Can you work these out from the model? Positions are in its coordinate system, mm. A direction names the side the tool comes from. Round coordinates to 2 decimals unless told otherwise and drop trailing zeros. Loops run counter-clockwise (first coordinate to the right, second up) from the corner with the lowest first, then second, coordinate; pieces in that order, holes last. Notation, with made-up numbers: (11, 41.25) -> (29, 41.25) arc R8 ccw to (29, 46.25) -> close; hole circle Ø10 at (75, 32). An arc over 180 degrees is marked (long way). Use a Markdown table: item, result.
from build123d import *

# Parameters (mm, degrees)
SKETCH_1_W           = 27
SKETCH_1_H           = 9
EXTRUDE_1_DEPTH      = 10
SKETCH_4_W           = 5
SKETCH_4_H           = 10
EXTRUDE_4_DEPTH      = 6
SKETCH_5_W           = 22
SKETCH_5_H           = 10
CUT_EXTRUDE_1_DEPTH  = 2
CUT_EXTRUDE_2_DEPTH  = 22
FILLET_1_R           = 1
FILLET_2_R           = 1
SKETCH_8_W           = 10
SKETCH_8_H           = 20
EXTRUDE_5_DEPTH      = 8
FILLET_3_R           = 2
FILLET_4_R           = 2
EXTRUDE_6_DEPTH      = 3
SKETCH_11_W          = 10
SKETCH_11_H          = 2.149089289
CUT_EXTRUDE_5_DEPTH  = 29.70975444
FILLET_5_R           = 2
FILLET_6_R           = 2
SKETCH_14_R          = 1.5
CUT_EXTRUDE_6_DEPTH  = 24.547823679
SKETCH_15_R          = 1.5
EXTRUDE_7_DEPTH      = 10
SKETCH_18_R          = 1.5
EXTRUDE_9_DEPTH      = 10
SKETCH_17_R          = 1.5
CUT_EXTRUDE_7_DEPTH  = 24.547823679
SKETCH_19_R          = 1.5
CUT_EXTRUDE_8_DEPTH  = 24.547823679
CUT_EXTRUDE_9_DEPTH  = 22
SKETCH_23_W          = 10
SKETCH_23_H          = 10
EXTRUDE_10_DEPTH     = 5
SKETCH_24_W          = 3.25
SKETCH_24_H          = 1.25
CUT_EXTRUDE_11_DEPTH = 4
CUT_EXTRUDE_12_DEPTH = 6.25
FILLET_7_R           = 2.5
FILLET_8_R           = 1
SKETCH_26_R          = 1.5
CUT_EXTRUDE_13_DEPTH = 35.383862494
SKETCH_27_R          = 1.75
CUT_EXTRUDE_14_DEPTH = 25.989997999
SKETCH_28_R          = 1.75
CUT_EXTRUDE_15_DEPTH = 35.383862494


with BuildPart() as part:
    # Эскиз1 → Бобышка-Вытянуть1 (new body)
    with BuildSketch(Plane.XY):
        Rectangle(SKETCH_1_W, SKETCH_1_H)
    extrude(amount=EXTRUDE_1_DEPTH)

    # Эскиз4 → Бобышка-Вытянуть4 (add)
    with BuildSketch(Plane(origin=(0, 4.5, 0), x_dir=(1, 0, 0), z_dir=(0, 1, 0))):
        with Locations((-11, -5)):
            Rectangle(SKETCH_4_W, SKETCH_4_H)
    extrude(amount=EXTRUDE_4_DEPTH)

    # Эскиз5 → Вырез-Вытянуть1 (cut)
    with BuildSketch(Plane(origin=(0, 4.5, 0), x_dir=(1, 0, 0), z_dir=(0, 1, 0))):
        with Locations((2.5, -5)):
            Rectangle(SKETCH_5_W, SKETCH_5_H)
    extrude(amount=-CUT_EXTRUDE_1_DEPTH, mode=Mode.SUBTRACT)

    # Эскиз6 → Вырез-Вытянуть2 (cut)
    with BuildSketch(Plane(origin=(13.5, 0, 0), x_dir=(0, 0, -1), z_dir=(1, 0, 0))):
        Polygon((-1.5, 2.5), (-8.5, 2.5), (-5, 0), align=None)
    extrude(amount=-CUT_EXTRUDE_2_DEPTH, mode=Mode.SUBTRACT)

    # Скругление1
    fillet_1_edges = [part.edges().sort_by_distance(p)[0] for p in [
        (-11, 10.5, 10),
    ]]
    fillet(fillet_1_edges, radius=FILLET_1_R)

    # Скругление2
    fillet_2_edges = [part.edges().sort_by_distance(p)[0] for p in [
        (-11, 10.5, 0),
    ]]
    fillet(fillet_2_edges, radius=FILLET_2_R)

    # Эскиз8 → Бобышка-Вытянуть5 (add)
    with BuildSketch(Plane.ZY.offset(13.5)):
        with Locations((5, 5.5)):
            Rectangle(SKETCH_8_W, SKETCH_8_H)
    extrude(amount=-EXTRUDE_5_DEPTH)

    # Скругление3
    fillet_3_edges = [part.edges().sort_by_distance(p)[0] for p in [
        (-9.5, 15.5, 10),
    ]]
    fillet(fillet_3_edges, radius=FILLET_3_R)

    # Скругление4
    fillet_4_edges = [part.edges().sort_by_distance(p)[0] for p in [
        (-9.5, 15.5, 0),
    ]]
    fillet(fillet_4_edges, radius=FILLET_4_R)

    # Эскиз9 → Бобышка-Вытянуть6 (add)
    with BuildSketch(Plane(origin=(13.5, 0, 0), x_dir=(0, 0, -1), z_dir=(1, 0, 0))):
        Polygon((-10, -4.5), (-10, 2.5), (-8.5, 2.5), (-5, 0), (-1.5, 2.5), (0, 2.5), (0, -4.5), align=None)
    extrude(amount=EXTRUDE_6_DEPTH)

    # Эскиз11 → Вырез-Вытянуть5 (cut, through all)
    with BuildSketch(Plane(origin=(-5.5, 0, 0), x_dir=(0, 0, -1), z_dir=(1, 0, 0))):
        with Locations((-5, 14.574544645)):
            Rectangle(SKETCH_11_W, SKETCH_11_H)
    extrude(amount=-CUT_EXTRUDE_5_DEPTH, mode=Mode.SUBTRACT)

    # Скругление5
    fillet_5_edges = [part.edges().sort_by_distance(p)[0] for p in [
        (-9.5, 13.5, 10),
    ]]
    fillet(fillet_5_edges, radius=FILLET_5_R)

    # Скругление6
    fillet_6_edges = [part.edges().sort_by_distance(p)[0] for p in [
        (-9.5, 13.5, 0),
    ]]
    fillet(fillet_6_edges, radius=FILLET_6_R)

    # Эскиз14 → Вырез-Вытянуть6 (cut, through all)
    with BuildSketch(Plane.XY.offset(10)):
        with Locations((-7.5, -1)):
            Circle(SKETCH_14_R)
        with Locations((10.5, -1)):
            Circle(SKETCH_14_R)
    extrude(amount=-CUT_EXTRUDE_6_DEPTH, mode=Mode.SUBTRACT)

    # Эскиз15 → Бобышка-Вытянуть7 (add, through all)
    with BuildSketch(Plane.XY.offset(10)):
        with Locations((10.5, -1)):
            Circle(SKETCH_15_R)
    extrude(amount=-EXTRUDE_7_DEPTH)

    # Эскиз18 → Бобышка-Вытянуть9 (add, through all)
    with BuildSketch(Plane.XY.offset(10)):
        with Locations((-7.5, -1)):
            Circle(SKETCH_18_R)
    extrude(amount=-EXTRUDE_9_DEPTH)

    # Эскиз17 → Вырез-Вытянуть7 (cut, through all)
    with BuildSketch(Plane.XY.offset(10)):
        with Locations((-7.5, -2)):
            Circle(SKETCH_17_R)
    extrude(amount=-CUT_EXTRUDE_7_DEPTH, mode=Mode.SUBTRACT)

    # Эскиз19 → Вырез-Вытянуть8 (cut, through all)
    with BuildSketch(Plane.XY.offset(10)):
        with Locations((10.5, -2)):
            Circle(SKETCH_19_R)
    extrude(amount=-CUT_EXTRUDE_8_DEPTH, mode=Mode.SUBTRACT)

    # Эскиз20 → Вырез-Вытянуть9 (cut)
    with BuildSketch(Plane(origin=(16.5, 0, 0), x_dir=(0, 0, -1), z_dir=(1, 0, 0))):
        Polygon((-8.5, 2.5), (-5, 0), (-1.5, 2.5), align=None)
    extrude(amount=-CUT_EXTRUDE_9_DEPTH, mode=Mode.SUBTRACT)

    # Эскиз23 → Бобышка-Вытянуть10 (add)
    with BuildSketch(Plane.ZY.offset(13.5)):
        with Locations((5, 0.5)):
            Rectangle(SKETCH_23_W, SKETCH_23_H)
    extrude(amount=EXTRUDE_10_DEPTH)

    # Эскиз24 → Вырез-Вытянуть11 (cut)
    with BuildSketch(Plane.ZY.offset(18.5)):
        with Locations((3.375, 1.125)):
            Rectangle(SKETCH_24_W, SKETCH_24_H)
        with Locations((6.625, 1.125)):
            Rectangle(SKETCH_24_W, SKETCH_24_H)
        with Locations((3.375, -0.125)):
            Rectangle(SKETCH_24_W, SKETCH_24_H)
        with Locations((6.625, -0.125)):
            Rectangle(SKETCH_24_W, SKETCH_24_H)
    extrude(amount=-CUT_EXTRUDE_11_DEPTH, mode=Mode.SUBTRACT)

    # Эскиз25 → Вырез-Вытянуть12 (cut)
    with BuildSketch(Plane(origin=(0, 5.5, 0), x_dir=(1, 0, 0), z_dir=(0, 1, 0))):
        Polygon((-13.5, -5), (-13.5, -1.75), (-16, -1.75), (-16, -8.25), (-13.5, -8.25), align=None)
    extrude(amount=-CUT_EXTRUDE_12_DEPTH, mode=Mode.SUBTRACT)

    # Скругление7
    fillet_7_edges = [part.edges().sort_by_distance(p)[0] for p in [
        (-13.5, 5.5, 9.125),
        (-13.5, 5.5, 0.875),
    ]]
    fillet(fillet_7_edges, radius=FILLET_7_R)

    # Скругление8
    fillet_8_edges = [part.edges().sort_by_distance(p)[0] for p in [
        (-18.5, 0.5, 0),
        (-18.5, -4.5, 5),
        (-18.5, 0.5, 10),
        (-18.5, 5.5, 5),
    ]]
    fillet(fillet_8_edges, radius=FILLET_8_R)

    # Эскиз26 → Вырез-Вытянуть13 (cut, through all)
    with BuildSketch(Plane.ZY.offset(13.5)):
        with Locations((5, 9.5)):
            Circle(SKETCH_26_R)
    extrude(amount=-CUT_EXTRUDE_13_DEPTH, mode=Mode.SUBTRACT)

    # Эскиз27 → Вырез-Вытянуть14 (cut, through all)
    with BuildSketch(Plane(origin=(0, 0, 0), x_dir=(-1, 0, 0), z_dir=(0, 0, -1))):
        with Locations((-10.5, -2)):
            Circle(SKETCH_27_R)
        with Locations((7.5, -2)):
            Circle(SKETCH_27_R)
    extrude(amount=-CUT_EXTRUDE_14_DEPTH, mode=Mode.SUBTRACT)

    # Эскиз28 → Вырез-Вытянуть15 (cut, through all)
    with BuildSketch(Plane.ZY.offset(13.5)):
        with Locations((5, 9.5)):
            Circle(SKETCH_28_R)
    extrude(amount=-CUT_EXTRUDE_15_DEPTH, mode=Mode.SUBTRACT)


solid = part.part
1. I want a section at C-C (z = 7.25). Please give me the cut outline in (x, y).
Answer sheet:
| item | result |
|---|---|
| outline | (-18.5, -3.5) arc R1 ccw to (-17.5, -4.5) -> (16.5, -4.5) -> (16.5, 1.61) -> (-5.5, 1.61) -> (-5.5, 13.5) -> (-13.5, 13.5) -> (-13.5, -0.75) -> (-18.5, -0.75) -> close; (-18.5, 1.75) -> (-16, 1.75) -> (-16, 5.5) -> (-17.5, 5.5) arc R1 ccw to (-18.5, 4.5) -> close; hole circle Ø3.5 at (-7.5, -2); hole circle Ø3.5 at (10.5, -2) |
2. I want a section at B-B (y = -2). Please give me the cut outline in (x, z).
Answer sheet:
| item | result |
|---|---|
| outline | (-18.5, 1) arc R1 ccw to (-17.5, 0) -> (-9.25, 0) -> (-9.25, 10) -> (-17.5, 10) arc R1 ccw to (-18.5, 9) -> close; (-5.75, 0) -> (8.75, 0) -> (8.75, 10) -> (-5.75, 10) -> close; (12.25, 0) -> (16.5, 0) -> (16.5, 10) -> (12.25, 10) -> close |
3. Which directions (+Z, -Z, +X, -X, +Y, -Y) give clear straight access to the entire face, cutting with the end or side of a thin tool? Please do faces 1 (the flat face through (5, 2.5, 1)), 2 (the flat face through (-16, -0.75, 5)), 3 (the flat face through (-16, 4, 5)).
Answer sheet:
| item | result |
|---|---|
| face 1 | +Z, -Z, +X, +Y |
| face 2 | -X |
| face 3 | +Y |
4. I want a section at A-A (x = -7.5). Please give me the cut outline in (y, z), plus the area to 3 significant figures.
Answer sheet:
| item | result |
|---|---|
| outline | (-4.5, 0) -> (-3.75, 0) -> (-3.75, 10) -> (-4.5, 10) -> close; (-0.25, 0) -> (11.5, 0) arc R2 ccw to (13.5, 2) -> (13.5, 8) arc R2 ccw to (11.5, 10) -> (-0.25, 10) -> close; hole circle Ø3.5 at (9.5, 5) |
| area | 134 mm² |
5. Will these pins go through, and if not, where does the flat tip stop? pin 1 Ø0.8 at (x, z) = (-16.5, 4) entering from +Y; pin 2 Ø4 at (y, z) = (9.5, 5) entering from +X; pin 3 Ø3 at (y, z) = (9.5, 7.5) entering from -X; pin 4 Ø3 at (x, y) = (-7.5, -2) entering from -Z.
Answer sheet:
| item | result |
|---|---|
| pin 1 | stops at y = 5.5 |
| pin 2 | stops at x = -5.5 |
| pin 3 | stops at x = -13.5 |
| pin 4 | passes through |
6. If we mould it in two halves opening along X, with no side actions, what happens to faces 4 (the flat face through (-17, 1.75, 5)), 5 (the cylindrical face through (-14.213, 6.252, 9.137)), 6 (the flat face through (-15, 2, 1.75))? For each: +X half, -X half, draft (parallel to the pull), parting line (faces both ways), or undercut.
Answer sheet:
| item | result |
|---|---|
| face 4 | draft |
| face 5 | -X half |
| face 6 | undercut |
7. I need wall thicknesses on line 1 (Y direction, x = -7.5, z = 5); line 2 (Y direction, x = -7.5, z = 7.5); line 3 (X direction, y = -1.25, z = 2.75). Which ranges of each line are inside material? Lowest first, please.
Answer sheet:
| item | result |
|---|---|
| line 1 | y = -4.5 to -3.75, -0.25 to 7.75, 11.25 to 13.5 |
| line 2 | y = -4.5 to -3.75, -0.25 to 13.5 |
| line 3 | x = -18.5 to -9.08, -5.92 to 8.92, 12.08 to 16.5 |
8. I want a section at D-D (x = 10.5). Please give me the cut outline in (y, z).
Answer sheet:
| item | result |
|---|---|
| outline | (-4.5, 0) -> (-3.75, 0) -> (-3.75, 10) -> (-4.5, 10) -> close; (-0.25, 0) -> (2.5, 0) -> (2.5, 1.5) -> (0, 5) -> (2.5, 8.5) -> (2.5, 10) -> (-0.25, 10) -> close |
